Design review of the part shown in the three views and the two pictorial views. Dimensions are in mm from the part's minimum x, y and z. A direction names the side the tool comes from. Coordinates: 2 decimals unless noted, no trailing zeros. Write each loop counter-clockwise with the first axis right and the second up, starting at its lowest first coordinate (ties: lowest second). Pieces come first, ordered by that corner, then holes.
Q1. Take a section at D-D, the plane z = 123. Write out the cut boundary in (x, y), plus the area to 3 significant figures.
Q2. Take a section at A-A, the plane x = 21.5. Write out the cut boundary in (y, z), plus the area to 3 significant figures.
Q3. For pin 1 Ø2 at (x, y) = (23.5, 2.5) entering from -Z; pin 2 Ø1.5 at (x, y) = (21, 5) entering from -Z, all flat-tipped, find the tip position at first contact; note any pin that passes through.
Q4. Take a section at C-C, the plane x = 3.5. Write out the cut boundary in (y, z).
Q5. Take a section at B-B, the plane y = 1.1. State how many separate pieces and enclosed holes the cut face has, plus the area to 3 significant figures.
Q6. For L1, parallel to X at y = 2.65, z = 44; L2, parallel to Z at x = 24.5, y = 2; L3, parallel to Y at x = 22, z = 142.5, list the stretches that pass through material, from the lowest coordinate up.
Q7. For the marked faces 1, 2 and 3, list the 3-axis set-ups (+Z, -Z, +X, -X, +Y, -Y) from which the entire face can be reached by the end or side of a thin tool; tool diameter is ignored.
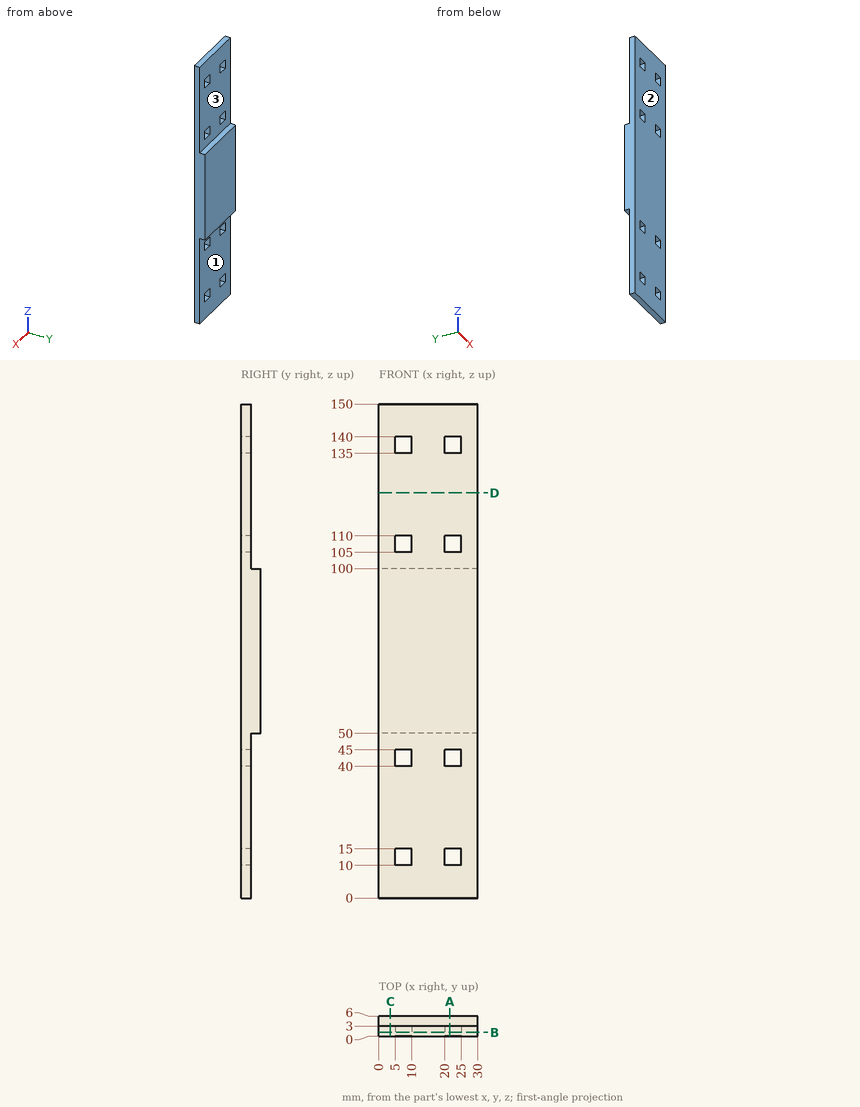
Responses:
1. outline: (0, 0) - (30, 0) - (30, 3) - (0, 3) - close
1. area: 90.0 mm2
2. outline: (0, 0) - (3, 0) - (3, 10) - (0, 10) - close; (0, 15) - (3, 15) - (3, 40) - (0, 40) - close; (0, 45) - (3, 45) - (3, 50) - (6, 50) - (6, 100) - (3, 100) - (3, 105) - (0, 105) - close; (0, 110) - (3, 110) - (3, 135) - (0, 135) - close; (0, 140) - (3, 140) - (3, 150) - (0, 150) - close
2. area: 540 mm2
3. pin 1: stops at z = 0
3. pin 2: stops at z = 50
4. outline: (0, 0) - (3, 0) - (3, 50) - (6, 50) - (6, 100) - (3, 100) - (3, 150) - (0, 150) - close
5. separate pieces: 1
5. enclosed holes: 8
5. area: 4,300 mm2
6. L1: x = 0 to 5, 10 to 20, 25 to 30
6. L2: z = 0 to 10, 15 to 40, 45 to 105, 110 to 135, 140 to 150
6. L3: y = 0 to 3
7. face 1: -Z, +X, -X, +Y
7. face 2: +Z, -Z, +X, -X, -Y
7. face 3: +Z, +X, -X, +Y
